```python
from build123d import *

# Parameters (mm, degrees)
EXTRUDE_1_DEPTH     = 35
EXTRUDE_2_DEPTH     = 3.18
SKETCH_3_R          = 1.75
CUT_EXTRUDE_1_DEPTH = 39.18
SKETCH_4_R          = 1.75
CUT_EXTRUDE_2_DEPTH = 39.18
SKETCH_5_R          = 1.75
CUT_EXTRUDE_3_DEPTH = 71
EXTRUDE_3_DEPTH     = 115.49
EXTRUDE_7_DEPTH     = 24
SKETCH_11_R         = 25
CUT_EXTRUDE_4_DEPTH = 20.82
SKETCH_12_R         = 1.75
CUT_EXTRUDE_5_DEPTH = 39.18
SKETCH_13_R         = 1.75
CUT_EXTRUDE_6_DEPTH = 24


with BuildPart() as part:
    # 草图1 → 凸台-拉伸1 (new body)
    with BuildSketch(Plane.XY):
        with BuildLine():
            Line((-30, 0), (-30, -115.49))
            Line((-30, -115.49), (-35, -115.49))
            Line((-35, -115.49), (-35, 0))
            ThreePointArc((-35, 0), (0, 35), (35, 0))
            Line((35, 0), (35, -115.49))
            Line((35, -115.49), (30, -115.49))
            Line((30, -115.49), (30, 0))
            ThreePointArc((30, 0), (0, 30), (-30, 0))
        make_face()
    extrude(amount=EXTRUDE_1_DEPTH)

    # 草图2 → 凸台-拉伸2 (add)
    with BuildSketch(Plane.XY.offset(35)):
        with BuildLine():
            Line((-30, -115.49), (30, -115.49))
            Line((30, -115.49), (35, -115.49))
            Line((35, -115.49), (35, 0))
            ThreePointArc((35, 0), (0, 35), (-35, 0))
            Line((-35, 0), (-35, -115.49))
            Line((-35, -115.49), (-30, -115.49))
        make_face()
    extrude(amount=EXTRUDE_2_DEPTH)

    # 草图3 → 切除-拉伸1 (cut, through all)
    with BuildSketch(Plane(origin=(0, 0, 0), x_dir=(-1, 0, 0), z_dir=(0, 0, -1))):
        with Locations((-26.795, -112.09)):
            Circle(SKETCH_3_R)
        with Locations((26.795, -112.09)):
            Circle(SKETCH_3_R)
    extrude(amount=-CUT_EXTRUDE_1_DEPTH, mode=Mode.SUBTRACT)

    # 草图4 → 切除-拉伸2 (cut, through all)
    with BuildSketch(Plane(origin=(0, 0, 0), x_dir=(-1, 0, 0), z_dir=(0, 0, -1))):
        with Locations((-26.795, -55.49)):
            Circle(SKETCH_4_R)
        with Locations((26.795, -55.49)):
            Circle(SKETCH_4_R)
    extrude(amount=-CUT_EXTRUDE_2_DEPTH, mode=Mode.SUBTRACT)

    # 草图5 → 切除-拉伸3 (cut, through all)
    with BuildSketch(Plane(origin=(35, 0, 0), x_dir=(0, 0, -1), z_dir=(1, 0, 0))):
        with Locations((-4.61, -19.28)):
            Circle(SKETCH_5_R)
    extrude(amount=-CUT_EXTRUDE_3_DEPTH, mode=Mode.SUBTRACT)

    # 草图6 → 凸台-拉伸3 (add)
    with BuildSketch(Plane.XZ.offset(115.49)):
        Polygon((30, 0), (35, 0), (35, 38.18), (-35, 38.18), (-35, 0), (-30, 0), (-30, 35), (30, 35), align=None)
    extrude(amount=EXTRUDE_3_DEPTH)

    # 草图10 → 凸台-拉伸7 (add)
    with BuildSketch(Plane.XY.offset(38.18)):
        with BuildLine():
            Line((35, -230.98), (-35, -230.98))
            ThreePointArc((-35, -230.98), (0, -265.98), (35, -230.98))
        make_face()
    extrude(amount=-EXTRUDE_7_DEPTH)

    # 草图11 → 切除-拉伸4 (cut)
    with BuildSketch(Plane(origin=(0, 0, 14.18), x_dir=(-1, 0, 0), z_dir=(0, 0, -1))):
        with Locations((0, -230.98)):
            Circle(SKETCH_11_R)
    extrude(amount=-CUT_EXTRUDE_4_DEPTH, mode=Mode.SUBTRACT)

    # 草图12 → 切除-拉伸5 (cut, through all)
    with BuildSketch(Plane.XY.offset(38.18)):
        with Locations((26.795, -119.23)):
            Circle(SKETCH_12_R)
        with Locations((-26.795, -119.23)):
            Circle(SKETCH_12_R)
    extrude(amount=-CUT_EXTRUDE_5_DEPTH, mode=Mode.SUBTRACT)

    # 草图13 → 切除-拉伸6 (cut)
    with BuildSketch(Plane.XY.offset(38.18)):
        with Locations((-26.795, -175.86)):
            Circle(SKETCH_13_R)
        with Locations((26.795, -175.86)):
            Circle(SKETCH_13_R)
    extrude(amount=-CUT_EXTRUDE_6_DEPTH, mode=Mode.SUBTRACT)


solid = part.part
```
The model under review builds one solid part; all positions refer to its coordinate system, in mm. A direction names the side the tool comes from. Round coordinates to 2 decimals unless told otherwise and drop trailing zeros. Order: outer loops, then holes, each group sorted by start corner. A loop starts at its lowest first (then second) coordinate and runs counter-clockwise, first axis right, second up.
(1) Take a section at C-C, the plane y = -205.5. State the section outline as (x, z) points.
Working result:
outline: (-35, 0) - (-30, 0) - (-30, 35) - (30, 35) - (30, 0) - (35, 0) - (35, 38.18) - (-35, 38.18) - close
(2) Take a section at A-A, the plane z = 27.5. State the section outline as (x, y) points.
Working result:
outline: (-35, -230.98) arc R35 ccw to (35, -230.98) - (35, 0) arc R35 ccw to (-35, 0) - close; hole (-30, -230.98) - (-25, -230.98) arc R25 ccw to (25, -230.98) - (30, -230.98) - (30, 0) arc R30 ccw to (-30, 0) - close
(3) Tool access review of faces 1 (the face through (35, -114, 19)), 2 (the face through (-33, -230.98, 7)), 3 (the face through (30, -114, 18)): name each direction out of +Z, -Z, +X, -X, +Y, -Y from which nothing blocks a thin tool from reaching the whole face with its end or side.
Working result:
face 1: +Z, -Z, +X, +Y, -Y
face 2: -Z, +X, -X, -Y
face 3: -Z
(4) Mouldability with a two-part tool opening along X and no side actions: class faces 4 (the face through (0.77, 34.99, 18.82)), 5 (the face through (31, -88, 0)), 6 (the face through (-30, -114, 17)) as released by +X, released by -X, zero draft, split by the parting line, or undercut.
Working result:
face 4: split by the parting line
face 5: zero draft
face 6: undercut
(5) For P1, Ø2, axis at x = 26.795, y = -119.23, coming from the +Z side; P2, Ø1.5, axis at x = -33.5, z = 8, coming from the -Y side; P3, Ø2, axis at x = 20.5, z = 13, coming from the -Y side; P4, Ø2.5, axis at x = 27, z = 25, coming from the +Y side, all flat-tipped, find the tip position at first contact; note any pin that passes through.
Working result:
P1: passes through
P2: stops at y = -230.98
P3: stops at y = 20.92
P4: stops at y = 23.71
(6) Wall thickness on L1, parallel to X at y = -43, z = 2.5; L2, parallel to Y at x = -0.5, z = 31 (3 decimals); L3, parallel to X at y = -55, z = 37 (3 decimals): over which ranges is each line inside the solid? List them lowest first.
Working result:
L1: x = -35 to -30, 30 to 35
L2: y = -265.976 to -255.975, 29.996 to 34.996
L3: x = -35 to -28.475, -25.115 to 25.115, 28.475 to 35
(7) Take a section at B-B, the plane x = 0. State the section outline as (y, z) points.
Working result:
outline: (-265.98, 14.18) - (-255.98, 14.18) - (-255.98, 35) - (30, 35) - (30, 0) - (35, 0) - (35, 38.18) - (-265.98, 38.18) - close
